The listing builds one solid part. Answer for the finished solid, in the listing's coordinates (mm). Face numbers are marked on the shaded views. A direction names the side the tool comes from. Give positions to 0.01 mm unless a question says otherwise; leave off trailing zeros. Loops run counter-clockwise (first coordinate to the right, second up) from the corner with the lowest first, then second, coordinate; pieces in that order, holes last.
Item 1: Section B-B, the plane x = -16 is taken. Give the number of separate pieces and of enclosed holes in the cut face, and give its area (3 significant figures).
Item 2: Consider line 1 along Z through (x, y) = (-14.25, 10.5); line 2 along X through (y, z) = (6.5, 15.25); line 3 along Y through (x, z) = (-4.2, 8). Determine where each line is inside the solid, lowest interval first.
Item 3: The mould has two halves that part along Z. Classify the marked faces 6, 7 and 8: pulls with the +Z half, pulls with the -Z half, needs draft (parallel to the pull), parting line crosses it, or undercut.
Item 4: A tool of negligible diameter and unlimited length cuts with its end or side. For the marked faces 1, 2, 3, 4 and 5, from which of +Z, -Z, +X, -X, +Y, -Y can it reach the whole face along a straight path? Write none if from no direction.
Item 5: Section C-C, the plane y = 13 is taken. Give the vertices of the cut face in (x, z).
Item 6: Each of these flat-tipped pins is pushed along its axis until it touches: pin 1 Ø3.5 at (y, z) = (8, 7) entering from -X; pin 2 Ø2.5 at (x, y) = (-16, 7.5) entering from -Z; pin 3 Ø3.5 at (y, z) = (7.5, 8) entering from +X. Where does it stop, or does it pass through?
Item 7: Section A-A, the plane z = 15.25 is taken. Give the vertices of the cut face in (x, y) (1 decimal).
from build123d import *

# Parameters (mm, degrees)
SKETCH1_W                = 22
SKETCH1_H                = 15
BOSS_EXTRUDE1_DEPTH      = 16
SKETCH2_R                = 1.5
CUT_EXTRUDE1_DEPTH       = 32.064449134
CUT_EXTRUDE2_DEPTH       = 5
CUT_EXTRUDE2_DEPTH_BACK  = 5
SKETCH3_R                = 10
SKETCH3_R_2              = 2.5
SKETCH4_W                = 9
SKETCH4_H                = 15
CUT_EXTRUDE3_DEPTH       = 15
SKETCH10_R               = 1.5
CUT_EXTRUDE5_DEPTH       = 32.064449134
SKETCH11_R               = 3.15
CUT_EXTRUDE6_DEPTH       = 1.45
CUT_EXTRUDE6_DRAFT       = -45
CUT_EXTRUDE8_DEPTH       = 2.5
FILLET1_R                = 5
FILLET2_R                = 0.5
SKETCH9_R                = 3.15
CUT_EXTRUDE10_DEPTH      = 1.45
CUT_EXTRUDE10_DRAFT      = -45
CUT_EXTRUDE12_DEPTH      = 1
CUT_EXTRUDE12_DEPTH_BACK = 2.5


with BuildPart() as part:
    # Sketch1 → Boss-Extrude1 (new body)
    with BuildSketch(Plane.XY):
        with Locations((-11, 7.5)):
            Rectangle(SKETCH1_W, SKETCH1_H)
    extrude(amount=BOSS_EXTRUDE1_DEPTH)

    # Sketch2 → Cut-Extrude1 (cut, through all)
    with BuildSketch(Plane.XY.offset(16)):
        with Locations((-17, 7.5)):
            Circle(SKETCH2_R)
    extrude(amount=-CUT_EXTRUDE1_DEPTH, mode=Mode.SUBTRACT)

    # Sketch3 → Cut-Extrude2 (cut, two sides: drawn at the far end of the back side and taken through both)
    with BuildSketch(Plane.XY.offset(8).offset(-CUT_EXTRUDE2_DEPTH_BACK)):
        with Locations((-17, 7.5)):
            Circle(SKETCH3_R)
        with Locations((-17, 7.5)):
            Circle(SKETCH3_R_2, mode=Mode.SUBTRACT)
    extrude(amount=CUT_EXTRUDE2_DEPTH + CUT_EXTRUDE2_DEPTH_BACK, mode=Mode.SUBTRACT)

    # Sketch4 → Cut-Extrude3 (cut)
    with BuildSketch(Plane.ZY.offset(22)):
        with Locations((8, 7.5)):
            Rectangle(SKETCH4_W, SKETCH4_H)
    extrude(amount=-CUT_EXTRUDE3_DEPTH, mode=Mode.SUBTRACT)

    # Sketch10 → Cut-Extrude5 (cut, through all)
    with BuildSketch(Plane(origin=(0, 0, 0), x_dir=(0, 0, -1), z_dir=(1, 0, 0))):
        with Locations((-8, 7.5)):
            Circle(SKETCH10_R)
    extrude(amount=-CUT_EXTRUDE5_DEPTH, mode=Mode.SUBTRACT)


with BuildPart() as cut_extrude6_tool:
    # Sketch11 → Cut-Extrude6 (with draft: the straight prism first)
    with BuildSketch(Plane.ZY.offset(7)):
        with Locations((8, 7.5)):
            Circle(SKETCH11_R)
    extrude(amount=-CUT_EXTRUDE6_DEPTH)
    # Cut-Extrude6: the draft: its side faces are tilted about the plane it starts from
    cut_extrude6_sides = [cut_extrude6_tool.faces().sort_by_distance(p)[0] for p in [
        (-6.275, 7.5, 4.85),
    ]]
    draft(cut_extrude6_sides, Plane.ZY.offset(7), CUT_EXTRUDE6_DRAFT)


with BuildPart() as part_1:
    add(part.part)

    # Cut-Extrude6: cut by cut_extrude6_tool
    add(cut_extrude6_tool.part, mode=Mode.SUBTRACT)

    # Sketch13 → Cut-Extrude8 (cut)
    with BuildSketch(Plane(origin=(0, 0, 0), x_dir=(0, 0, -1), z_dir=(1, 0, 0))):
        Polygon((-5.250369343, 9.0875), (-8, 10.675), (-10.749630657, 9.0875), (-10.749630657, 5.9125), (-8, 4.325), (-5.250369343, 5.9125), align=None)
    extrude(amount=-CUT_EXTRUDE8_DEPTH, mode=Mode.SUBTRACT)

    # Fillet1
    fillet1_edges = [part_1.edges().sort_by_distance(p)[0] for p in [
        (-22, 0, 1.5),
        (-22, 15, 1.5),
        (-22, 0, 14.5),
        (-22, 15, 14.5),
    ]]
    fillet(fillet1_edges, radius=FILLET1_R)

    # Fillet2
    fillet2_edges = [part_1.edges().sort_by_distance(p)[0] for p in [
        (0, 7.5, 16),
        (-7, 15, 8),
        (-7, 0, 8),
        (0, 7.5, 0),
        (0, 0, 8),
        (0, 15, 8),
    ]]
    fillet(fillet2_edges, radius=FILLET2_R)


with BuildPart() as cut_extrude10_tool:
    # Sketch9 → Cut-Extrude10 (with draft: the straight prism first)
    with BuildSketch(Plane(origin=(0, 0, 0), x_dir=(-1, 0, 0), z_dir=(0, 0, -1))):
        with Locations((17, 7.5)):
            Circle(SKETCH9_R)
    extrude(amount=-CUT_EXTRUDE10_DEPTH)
    # Cut-Extrude10: the draft: its side faces are tilted about the plane it starts from
    cut_extrude10_sides = [cut_extrude10_tool.faces().sort_by_distance(p)[0] for p in [
        (-13.85, 7.5, 0.725),
    ]]
    draft(cut_extrude10_sides, Plane(origin=(0, 0, 0), x_dir=(-1, 0, 0), z_dir=(0, 0, -1)), CUT_EXTRUDE10_DRAFT)


with BuildPart() as part_2:
    add(part_1.part)

    # Cut-Extrude10: cut by cut_extrude10_tool
    add(cut_extrude10_tool.part, mode=Mode.SUBTRACT)

    # Sketch12 → Cut-Extrude12 (cut, two sides: drawn at the far end of the back side and taken through both)
    with BuildSketch(Plane.XY.offset(16).offset(-CUT_EXTRUDE12_DEPTH_BACK)):
        Polygon((-14.250369343, 9.0875), (-17, 10.675), (-19.749630657, 9.0875), (-19.749630657, 5.9125), (-17, 4.325), (-14.250369343, 5.9125), align=None)
    extrude(amount=CUT_EXTRUDE12_DEPTH + CUT_EXTRUDE12_DEPTH_BACK, mode=Mode.SUBTRACT)


solid = part_2.part
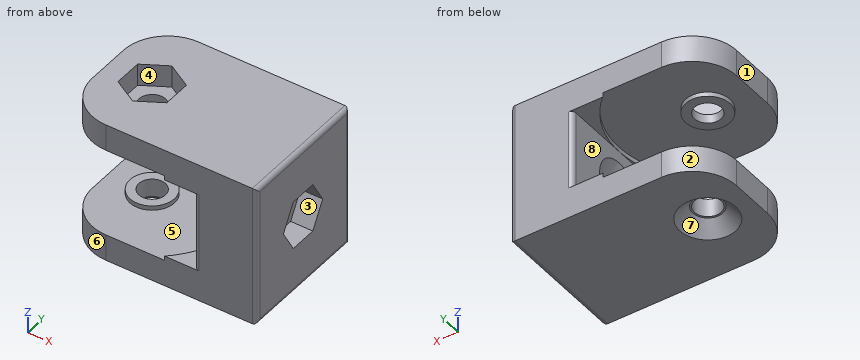
Worked answers:
1. separate pieces: 4
1. enclosed holes: 0
1. area: 68.4 mm2
2. line 1: z = 0 to 3, 13 to 16
2. line 2: x = -22 to -19.75, -14.25 to 0
2. line 3: y = 0 to 6, 9 to 15
3. face 6: needs draft
3. face 7: pulls with the -Z half
3. face 8: undercut
4. face 1: +Z, -Z, -X, +Y, -Y
4. face 2: +Z, -Z, -X, +Y
4. face 3: +X
4. face 4: +Z
4. face 5: none
5. outline: (-21, 0) - (-0.5, 0) arc R0.5 ccw to (0, 0.5) - (0, 15.5) arc R0.5 ccw to (-0.5, 16) - (-21, 16) - (-21, 13) - (-8.65, 13) - (-8.65, 12.5) - (-7, 12.5) - (-7, 3.5) - (-8.65, 3.5) - (-8.65, 3) - (-21, 3) - close
6. pin 1: stops at x = -6.72
6. pin 2: stops at z = 0.9
6. pin 3: stops at x = -2.5
7. outline: (-22, 5) arc R5 ccw to (-17, 0) - (-0.5, 0) arc R0.5 ccw to (0, 0.5) - (0, 14.5) arc R0.5 ccw to (-0.5, 15) - (-17, 15) arc R5 ccw to (-22, 10) - close; hole (-19.7, 5.9) - (-17, 4.3) - (-14.3, 5.9) - (-14.3, 9.1) - (-17, 10.7) - (-19.7, 9.1) - close
